Check sheet for the modelled part. Datum: model origin and axes. Units: mm. A direction names the side the tool comes from. Give positions to 0.01 mm unless a question says otherwise; leave off trailing zeros. Order: outer loops, then holes, each group sorted by start corner. A loop starts at its lowest first (then second) coordinate and runs counter-clockwise, first axis right, second up.
Item 1: Release check for a two-part mould opening along X. For faces 1 (the flat face through (27, 39, 4)), 2 (the flat face through (56, 50, 4)), 3 (the flat face through (49, 31, 7.5)), 4 (the flat face through (9, 31, 4)) record: released by +X, released by -X, zero draft, split by the parting line, or undercut.
Item 2: Material ranges on line 1 along X through (y, z) = (36, 3.5); line 2 along X through (y, z) = (54.5, 4); line 3 along Y through (x, z) = (50.5, 1.25), recorded low to high.
Item 3: Sectioned sample at D-D on y = 11. Record the boundary of the cut face in (x, z).
Item 4: Access from +Z, -Z, +X, -X, +Y, -Y to the whole of each face (thin tool, end or side, straight path). Record for faces 5 (the flat face through (33, 50, 4)), 6 (the flat face through (94, 28, 3)), 7 (the flat face through (19, 25, 4)), 8 (the flat face through (40, 36, 6)).
Item 5: Sectioned sample at B-B on x = 50. Record the boundary of the cut face in (y, z).
Item 6: Sectioned sample at C-C on z = 8.75. Record the boundary of the cut face in (x, y), and give its area (3 significant figures).
Item 7: Sectioned sample at A-A on y = 35. Record the boundary of the cut face in (x, z).
Item 8: Gauge pin test, flat ends, axial feed: P1, Ø2, axis at x = 22, z = 4.5, coming from the +Y side; P2, Ø0.8, axis at x = 39, z = 5.5, coming from the -Y side; P3, Ø5, axis at y = 40, z = 5.5, coming from the +X side. Record the tip position at first contact, or that the pin passes through.
Autodesk Fusion 360 part; units mm, degrees
sketch "elephant sketch" plane through (0, 0, 0) normal (0, 0, 1) x (1, 0, 0)
  line L0 (5, 40) -> (5, 33)
  line L1 (5, 33) -> (9, 33)
  line L2 (9, 33) -> (9, 29)
  line L3 (9, 29) -> (13, 29)
  line L4 (13, 29) -> (13, 25)
  line L5 (13, 25) -> (25, 25)
  line L6 (25, 25) -> (25, 21)
  line L7 (25, 21) -> (36, 21)
  line L8 (36, 21) -> (36, 17)
  line L9 (36, 17) -> (52, 17)
  line L10 (52, 17) -> (52, 13)
  line L11 (52, 13) -> (47, 13)
  line L12 (47, 13) -> (47, 6)
  line L13 (47, 6) -> (59, 6)
  line L14 (59, 6) -> (59, 9.5)
  line L15 (59, 9.5) -> (63, 9.5)
  line L16 (63, 9.5) -> (63, 13)
  line L17 (63, 13) -> (78, 13)
  line L18 (78, 13) -> (78, 6)
  line L19 (78, 6) -> (90, 6)
  line L20 (90, 6) -> (90, 9.5)
  line L21 (90, 9.5) -> (94, 9.5)
  line L22 (94, 9.5) -> (94, 28)
  line L23 (94, 28) -> (90, 28)
  line L24 (90, 28) -> (90, 24)
  line L25 (90, 24) -> (86, 24)
  line L26 (86, 24) -> (86, 20)
  line L27 (86, 20) -> (67, 20)
  line L28 (67, 20) -> (67, 24)
  line L29 (67, 24) -> (63, 24)
  line L30 (63, 24) -> (63, 28)
  line L31 (63, 28) -> (59, 28)
  line L32 (59, 28) -> (59, 50)
  line L33 (59, 50) -> (52, 50)
  line L34 (52, 50) -> (52, 55)
  line L35 (52, 55) -> (41, 55)
  line L36 (41, 55) -> (41, 51)
  line L37 (41, 51) -> (33, 51)
  line L38 (33, 51) -> (33, 48)
  line L39 (33, 48) -> (29, 48)
  line L40 (29, 48) -> (29, 39)
  line L41 (29, 39) -> (25, 39)
  line L42 (25, 39) -> (25, 33)
  line L43 (25, 33) -> (17, 33)
  line L44 (17, 33) -> (17, 37)
  line L45 (17, 37) -> (13, 37)
  line L46 (13, 37) -> (13, 40)
  line L47 (13, 40) -> (5, 40)
  line L48 (94, 28) -> (98, 28)
  line L49 (98, 28) -> (98, 32)
  line L50 (98, 32) -> (102, 32)
  line L51 (102, 32) -> (102, 24)
  line L52 (102, 24) -> (94, 24)
  line L53 (59, 50) -> (59, 54)
  line L54 (59, 54) -> (65, 54)
  line L55 (65, 54) -> (65, 58.7382)
  line L56 (65, 58.7382) -> (81.9319, 58.7382)
  line L57 (81.9319, 58.7382) -> (81.9319, 54)
  line L58 (81.9319, 54) -> (87.0128, 54)
  line L59 (87.0128, 54) -> (87.0128, 51.2757)
  line L60 (87.0128, 51.2757) -> (90, 51.2757)
  line L61 (90, 51.2757) -> (90, 28)
  line L62 (36.8391, 40.0538) -> (36.8391, 32.8575)
  line L63 (36.8391, 32.8575) -> (40, 32.8575)
  line L64 (40, 32.8575) -> (40, 40.0538)
  line L65 (40, 40.0538) -> (36.8391, 40.0538)
  line L66 (71, 57) -> (75, 57)
  line L67 (75, 57) -> (75, 55)
  line L68 (75, 55) -> (70, 55)
  line L69 (70, 55) -> (70, 57)
  line L70 (70, 57) -> (71, 57)
extrude "Extrude1" add sketch "elephant sketch" along normal blind 7.5 contours L0 L1 L2 L3 L4 L5 L6 L7 L8 L9 L10 L11 L12 L13 L14 L15 L16 L17 L18 L19 L20 L21 L22 L23 L24 L25 L26 L27 L28 L29 L30 L31 L32 L33 L34 L35 L36 L37 L38 L39 L40 L41 L42 L43 L44 L45 L46 L47
extrude "Extrude2" add sketch "elephant sketch" along normal blind 10 contours L24 L25 L26 L27 L28 L29 L30 L31 L32 L53 L54 L55 L56 L57 L58 L59 L60 L61 | L66 L67 L68 L69 L70
extrude "Extrude3" add sketch "elephant sketch" along normal blind 5 contours L22 L48 L49 L50 L51 L52
extrude "Extrude4" add sketch "elephant sketch" along normal blind 5 contours L62 L63 L64 L65
extrude "Extrude5" cut sketch "elephant sketch" along normal blind 13 contours L66 L67 L68 L69 L70
Report:
1. face 1: undercut
1. face 2: undercut
1. face 3: zero draft
1. face 4: released by -X
2. line 1: x = 5 to 17, 25 to 90
2. line 2: x = 41 to 52, 65 to 81.93
2. line 3: y = 6 to 13, 17 to 55
3. outline: (47, 0) - (63, 0) - (63, 7.5) - (47, 7.5) - close; (78, 0) - (94, 0) - (94, 7.5) - (78, 7.5) - close
4. face 5: +Z, -Z, -X, +Y
4. face 6: +Z, -Z, +Y
4. face 7: +Z, -Z, -X, -Y
4. face 8: +Z
5. outline: (6, 0) - (13, 0) - (13, 7.5) - (6, 7.5) - close; (17, 0) - (55, 0) - (55, 7.5) - (17, 7.5) - close
6. outline: (59, 28) - (63, 28) - (63, 24) - (67, 24) - (67, 20) - (86, 20) - (86, 24) - (90, 24) - (90, 51.28) - (87.01, 51.28) - (87.01, 54) - (81.93, 54) - (81.93, 58.74) - (65, 58.74) - (65, 54) - (59, 54) - close; hole (70, 55) - (75, 55) - (75, 57) - (70, 57) - close
6. area: 1,050 mm2
7. outline: (5, 0) - (17, 0) - (17, 7.5) - (5, 7.5) - close; (25, 0) - (90, 0) - (90, 10) - (59, 10) - (59, 7.5) - (40, 7.5) - (40, 5) - (36.84, 5) - (36.84, 7.5) - (25, 7.5) - close
8. P1: stops at y = 33
8. P2: stops at y = 17
8. P3: stops at x = 90
